For this review, take the finished solid that the model builds, in its own axes (mm). Give positions to 0.01 mm unless a question says otherwise; leave off trailing zeros. Order: outer loops, then holes, each group sorted by start corner. A loop starts at its lowest first (then second) coordinate and runs counter-clockwise, first axis right, second up.
from build123d import *

# Parameters (mm, degrees)
SKETCH1_R           = 9
SKETCH1_R_2         = 3
BOSS_EXTRUDE1_DEPTH = 9.5
FILLET1_R           = 2
FILLET2_R           = 2
SCALE1_SCALE        = 0.5


with BuildPart() as part:
    # Sketch1 → Boss-Extrude1 (new body)
    with BuildSketch(Plane.XY):
        Circle(SKETCH1_R)
        Circle(SKETCH1_R_2, mode=Mode.SUBTRACT)
    extrude(amount=BOSS_EXTRUDE1_DEPTH)

    # Fillet1
    fillet1_edges = [part.edges().sort_by_distance(p)[0] for p in [
        (-3, 0, 0),
        (-3, 0, 9.5),
    ]]
    fillet(fillet1_edges, radius=FILLET1_R)

    # Fillet2
    fillet2_edges = [part.edges().sort_by_distance(p)[0] for p in [
        (-9, 0, 0),
        (-9, 0, 9.5),
    ]]
    fillet(fillet2_edges, radius=FILLET2_R)


with BuildPart() as part_1:
    # Scale1: scaled about (0, 0, 0)
    add(part.part.scale(SCALE1_SCALE))


solid = part_1.part
1) We need section C-C on z = 0.4. Give the boundary of the cut face in (x, y).
Answer sheet:
outline: circle Ø8.6 at (0, 0); hole circle Ø3.4 at (0, 0)
2) Clearance check with flat-ended pins moving along their axes: pin 1 (3.5 mm diameter, centred on x = 0, y = 0, fed in from -Z); pin 2 (1 mm diameter, centred on y = 2.5, z = 0.5, fed in from +X). State where each tip first meets the part, or that it passes through.
Answer sheet:
pin 1: stops at z = 0.34
pin 2: stops at x = 3.96
3) To check wall thickness, follow line 1 (Y direction, x = 0, z = 1.65); line 2 (Y direction, x = 0, z = 0.4); line 3 (X direction, y = -1, z = 4). State the ranges of each line that lie inside material, in increasing order.
Answer sheet:
line 1: y = -4.5 to -1.5, 1.5 to 4.5
line 2: y = -4.3 to -1.7, 1.7 to 4.3
line 3: x = -4.35 to -1.16, 1.16 to 4.35
4) Draft analysis for pull direction Z (two halves, no side actions). For faces 1 (the face through (-0.59, 4.46, 2.36)), 2 (the face through (2, -2, 0)), 3 (the face through (2, -2, 4.75)), state which applies: +Z half, -Z half, draft (parallel to the pull), parting line (faces both ways), or undercut.
Answer sheet:
face 1: draft
face 2: -Z half
face 3: +Z half
5) We need section A-A on x = 0. Give the boundary of the cut face in (y, z), then the cut area to 3 significant figures.
Answer sheet:
outline: (-4.5, 1) arc R1 ccw to (-3.5, 0) - (-2.5, 0) arc R1 ccw to (-1.5, 1) - (-1.5, 3.75) arc R1 ccw to (-2.5, 4.75) - (-3.5, 4.75) arc R1 ccw to (-4.5, 3.75) - close; (1.5, 1) arc R1 ccw to (2.5, 0) - (3.5, 0) arc R1 ccw to (4.5, 1) - (4.5, 3.75) arc R1 ccw to (3.5, 4.75) - (2.5, 4.75) arc R1 ccw to (1.5, 3.75) - close
area: 26.8 mm2
6) We need section D-D on z = 1.65. Give the boundary of the cut face in (x, y).
Answer sheet:
outline: circle Ø9 at (0, 0); hole circle Ø3 at (0, 0)
